The figure shows three views and two pictorial views of one solid part (mm, origin at its lowest corner). Answer the questions. A direction names the side the tool comes from. Coordinates: 2 decimals unless noted, no trailing zeros. Loops run counter-clockwise (first coordinate to the right, second up) from the corner with the lowest first, then second, coordinate; pieces in that order, holes last. Notation, with made-up numbers: (-8, 40.25) -> (-2, 40.25) arc R24 cw to (-2, 55.25) -> close; hole circle Ø4 at (-37.5, -37). An arc over 180 degrees is marked (long way). Answer as a JSON object with one key per item and string values. Group by question number.
1) Section B-B, the plane z = 29 is taken. Give the vertices of the cut face in (x, y), plus the area to 3 significant figures.
2) Flat-ended cylindrical pins translate along their axes: P1, Ø7, axis at x = 16.5, z = 6, coming from the -Y side; P2, Ø1.5, axis at x = 3.5, y = 15.5, coming from the +Z side; P3, Ø3, axis at y = 12, z = 30, coming from the -X side. Find the tip coordinate at first contact, or state that the pin passes through.
3) Section C-C, the plane x = 16.5 is taken. Give the vertices of the cut face in (y, z) (1 decimal).
4) Consider probe 1 along X at (y, z) = (17.3, 29); probe 2 along Y at (x, z) = (8.5, 9); probe 3 along Z at (x, y) = (25, 7.75). Determine where each line is inside the solid, lowest interval first. Write a range as [from, to].
5) Which of the six approach directions +Z, -Z, +X, -X, +Y, -Y give full straight-line access (tool end or side, diameter ignored) to the marked faces 4, 5 and 6?
6) Determine the mould class of the marked faces 1, 2 and 3 for opening direction Y: released by +Y, released by -Y, zero draft, split by the parting line, or undercut.
7) Section D-D, the plane z = 7 is taken. Give the vertices of the cut face in (x, y) (1 decimal).
8) Section A-A, the plane y = 18 is taken. Give the vertices of the cut face in (x, z).
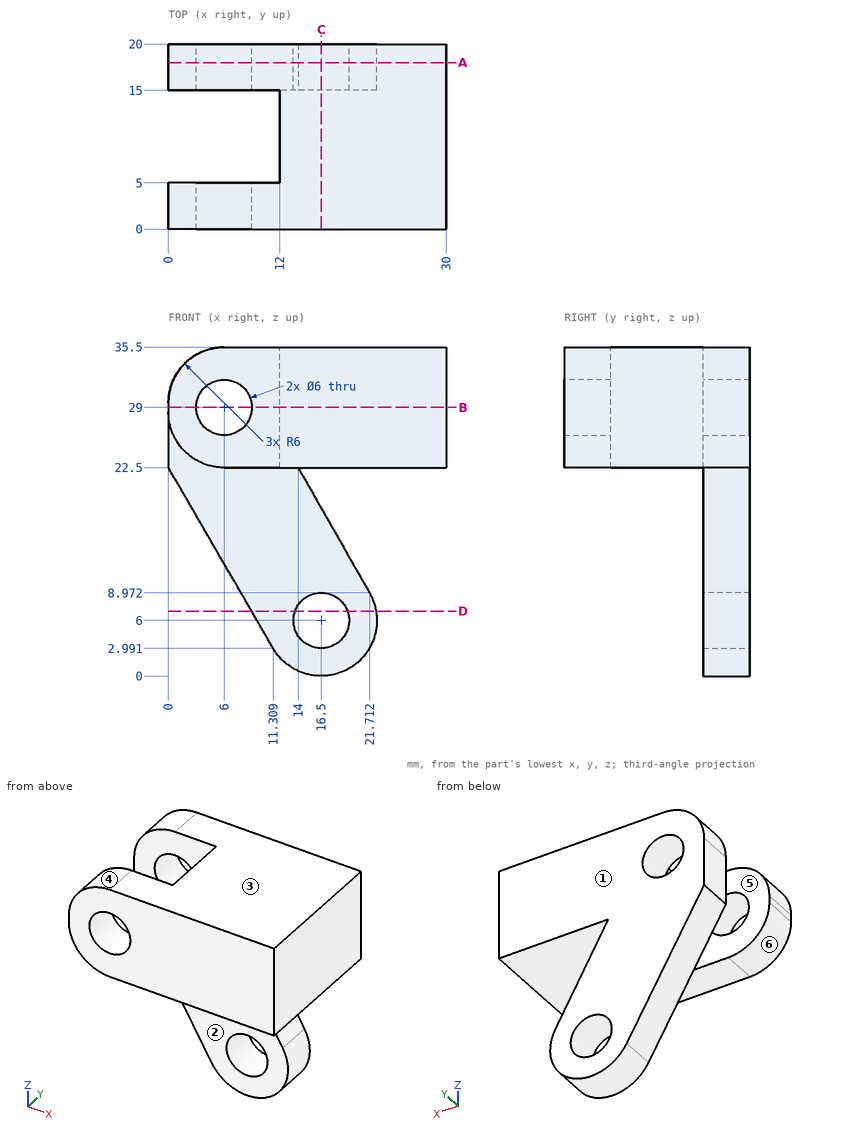
Determined:
{
 "1": {"outline": "(0, 0) -> (3, 0) -> (3, 5) -> (0, 5) -> close; (0, 15) -> (3, 15) -> (3, 20) -> (0, 20) -> close; (9, 0) -> (30, 0) -> (30, 20) -> (9, 20) -> (9, 15) -> (12, 15) -> (12, 5) -> (9, 5) -> close", "area": "420 mm²"},
 "2": {"P1": "y = 15", "P2": "z = 35.24", "P3": "x = 12"},
 "3": {"outline": "(0, 22.5) -> (20, 22.5) -> (20, 35.5) -> (0, 35.5) -> close; (15, 0) -> (20, 0) -> (20, 3) -> (15, 3) -> close; (15, 9) -> (20, 9) -> (20, 18.1) -> (15, 18.1) -> close"},
 "4": {"probe 1": "[0, 3], [9, 30]", "probe 2": "[15, 20]", "probe 3": "[22.5, 35.5]"},
 "5": {"face 4": "+Z, -X, +Y, -Y", "face 5": "+Z, -Z, -X", "face 6": "-Z, -X, -Y"},
 "6": {"face 1": "released by +Y", "face 2": "undercut", "face 3": "zero draft"},
 "7": {"outline": "(9, 15) -> (13.7, 15) -> (13.7, 20) -> (9, 20) -> close; (19.3, 15) -> (22.4, 15) -> (22.4, 20) -> (19.3, 20) -> close"},
 "8": {"outline": "(0, 22.5) -> (11.31, 2.99) arc R6 ccw to (21.71, 8.97) -> (14, 22.5) -> (30, 22.5) -> (30, 35.5) -> (6, 35.5) arc R6 ccw to (0, 29.5) -> close; hole circle Ø6 at (6, 29); hole circle Ø6 at (16.5, 6)"}
}
